Here's how the part is built. I have some questions about the finished solid (model axes, mm). Face numbers are marked on the shaded views. A direction names the side the tool comes from. Coordinates: 2 decimals unless noted, no trailing zeros. Order: outer loops, then holes, each group sorted by start corner. A loop starts at its lowest first (then second) coordinate and runs counter-clockwise, first axis right, second up.
```python
from build123d import *

# Parameters (mm, degrees)
SKIZZE3_R                       = 10.075
SCHNITT_LINEAR_AUSTRAGEN1_DEPTH = 34.526109228
SKIZZE4_R                       = 2.1
SCHNITT_LINEAR_AUSTRAGEN2_DEPTH = 34.526109228
VERRUNDUNG1_R                   = 3
FASE1_SIZE                      = 2


with BuildPart() as part:
    # Skizze2 → Rotation1 (revolve)
    with BuildSketch(Plane.XY, mode=Mode.PRIVATE) as rotation1_sk:
        Polygon((0, 0), (20, 0), (20, 5), (12.5, 5), (12.5, 18), (0, 18), align=None)
    revolve(rotation1_sk.sketch.rotate(Axis((0, 0, 0), (0, 1, 0)), 90), axis=Axis((0, 0, 0), (0, 1, 0)))

    # Skizze3 → Schnitt-Linear austragen1 (cut, through all)
    with BuildSketch(Plane(origin=(0, 18, 0), x_dir=(1, 0, 0), z_dir=(0, 1, 0))):
        with Locations(Location((0, 0, 0), (0, 0, 270))):
            Circle(SKIZZE3_R)
    extrude(amount=-SCHNITT_LINEAR_AUSTRAGEN1_DEPTH, mode=Mode.SUBTRACT)

    # Skizze4 → Schnitt-Linear austragen2 (cut, through all)
    with BuildSketch(Plane.XY):
        with Locations((0, 11.5)):
            Circle(SKIZZE4_R)
    extrude(amount=-SCHNITT_LINEAR_AUSTRAGEN2_DEPTH, mode=Mode.SUBTRACT)

    # Verrundung1
    verrundung1_edges = [part.edges().sort_by_distance(p)[0] for p in [
        (0, 5, 12.5),
    ]]
    fillet(verrundung1_edges, radius=VERRUNDUNG1_R)

    # Fase1
    fase1_edges = [part.edges().sort_by_distance(p)[0] for p in [
        (0, 0, -10.075),
    ]]
    chamfer(fase1_edges, length=FASE1_SIZE)


solid = part.part
```
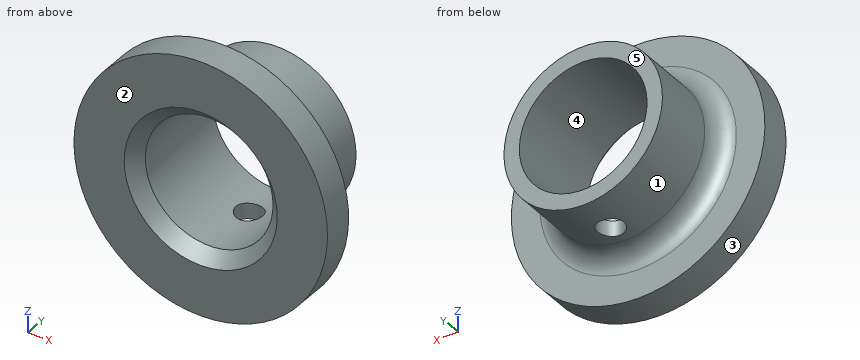
Q1. We'd pull the mould along X, two halves only. Please class the marked faces 3, 4 and 5: pulls with the +X half, pulls with the -X half, needs draft (parallel to the pull), parting line crosses it, or undercut.
Q2. If we section it at A-A on x = 0: Write out the boundary of the cut face in (y, z) (3 decimals), then the cut area to 3 significant figures.
Q3. If we section it at D-D on y = 15.75: Write out the boundary of the cut face in (x, z) (3 decimals), then the cut area to 3 significant figures.
Q4. If we section it at C-C on y = 3.25: Write out the boundary of the cut face in (x, z) (3 decimals), then the cut area to 3 significant figures.
Q5. For the marked faces 1 and 2, which set-ups out of +Z, -Z, +X, -X, +Y, -Y let a thin tool reach every point of the face, with its end or its side?
Q6. I need wall thicknesses on L1, parallel to X at y = 14.75, z = 0 (3 decimals); L2, parallel to X at y = 15, z = 6.5; L3, parallel to Z at x = -8, y = 1. Which ranges of each line are inside material? Lowest first, please.
Q7. Will these pins go through, and if not, where does the flat tip stop? pin 1 (5.5 mm diameter, centred on x = 0, y = 11.5, fed in from -Z); pin 2 (5 mm diameter, centred on x = 2, y = 10, fed in from +Z); pin 3 (1 mm diameter, centred on y = 7.5, z = 11, fed in from -X); pin 4 (12 mm diameter, centred on x = 8.5, z = 3.5, fed in from +Y).
Q8. If we section it at B-B on z = 0: Write out the boundary of the cut face in (x, y) (3 decimals), then the cut area to 3 significant figures.
Reply:
1. face 3: parting line crosses it
1. face 4: undercut
1. face 5: needs draft
2. outline: (0, -20) - (5, -20) - (5, -15.5) arc R3 cw to (8, -12.5) - (9.4, -12.5) - (9.4, -10.075) - (2, -10.075) - (0, -12.075) - close; (0, 12.075) - (2, 10.075) - (18, 10.075) - (18, 12.5) - (8, 12.5) arc R3 cw to (5, 15.5) - (5, 20) - (0, 20) - close; (13.6, -12.5) - (18, -12.5) - (18, -10.075) - (13.6, -10.075) - close
2. area: 152 mm2
3. outline: circle Ø25 at (0, 0); hole circle Ø20.15 at (0, 0)
3. area: 172 mm2
4. outline: circle Ø40 at (0, 0); hole circle Ø20.15 at (0, 0)
4. area: 938 mm2
5. face 1: +Y
5. face 2: +Z, -Z, +X, -X, -Y
6. L1: x = -12.5 to -10.075, 10.075 to 12.5
6. L2: x = -10.68 to -7.7, 7.7 to 10.68
6. L3: z = -18.33 to -7.66, 7.66 to 18.33
7. pin 1: stops at z = -12.5
7. pin 2: stops at z = 12.5
7. pin 3: stops at x = -6.88
7. pin 4: stops at y = 18
8. outline: (-20, 0) - (-12.075, 0) - (-10.075, 2) - (-10.075, 18) - (-12.5, 18) - (-12.5, 8) arc R3 cw to (-15.5, 5) - (-20, 5) - close; (10.075, 2) - (12.075, 0) - (20, 0) - (20, 5) - (15.5, 5) arc R3 cw to (12.5, 8) - (12.5, 18) - (10.075, 18) - close
8. area: 162 mm2
